Part model, mm, in its own coordinate system. Face numbers are marked on the shaded views. Round coordinates to 2 decimals unless told otherwise and drop trailing zeros. Write each loop counter-clockwise with the first axis right and the second up, starting at its lowest first coordinate (ties: lowest second). Pieces come first, ordered by that corner, then holes.
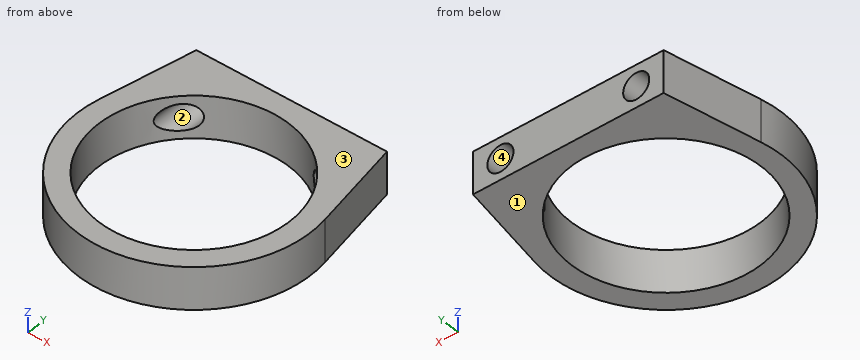
Autodesk Inventor part; units mm, degrees
ref_plane "YZ Plane" through (0, 0, 0) normal (1, 0, 0) x (0, 1, 0)
ref_plane "XZ Plane" through (0, 0, 0) normal (0, 1, 0) x (-1, 0, 0)
ref_plane "XY Plane" through (0, 0, 0) normal (0, 0, 1) x (1, 0, 0)
sketch "Sketch1" plane through (0, 0, 0) normal (0, 0, 1) x (1, 0, 0)
  circle A0 centre (0, 0) radius 9
  circle A1 centre (0, 0) radius 11
  line L0 (-9.125, 11) -> (9.125, 11)
  line L1 (0, 0) -> (0, 11) construction
  line L2 (-9.125, 11) -> (-10.8107, 2.0321)
  line L3 (9.125, 11) -> (10.8107, 2.0321)
  dimension "d0" = 18
  dimension "d1" = 22
  dimension "d2" = 18.25
extrude "Extrusion1" add sketch "Sketch1" along normal blind 4
sketch "Sketch2" plane through (-9.125, 11, 0) normal (0, 1, 0) x (1, 0, 0)
  line L0 (18.25, -4) -> (0, -4) construction
  line L1 (9.125, -4) -> (9.125, 0) construction
  line L2 (9.125, -2) -> (2.625, -2) construction
  line L3 (2.625, -2) -> (15.625, -2) construction
  circle A0 centre (2.625, -2) radius 1.25
  circle A1 centre (15.625, -2) radius 1.25
  dimension "d5" = 6.5
  dimension "d6" = 13
  dimension "d7" = 2.5
  dimension "d8" = 2.5
extrude "Extrusion2" cut sketch "Sketch2" against normal blind 11
thread "Thread1"
thread "Thread2"
equation "\"d6\" = 2 * d5"
properties part number "Tarot_12mm_Mount" material "Aluminum 6061"
Q1. Drop flat-ended pins along their axis: pin 1 (2 mm diameter, centred on x = -6.5, z = 2, fed in from -Y); pin 2 (12 mm diameter, centred on x = 5, y = -4, fed in from -Z). Give the stop position or say it passes through.
Values follow:
pin 1: stops at y = -9.53
pin 2: stops at z = 0
Q2. Cut at C-C on z = 1.6. Write the cut outline in (x, y) (3 decimals), plus the area to 3 significant figures.
Values follow:
outline: (-10.811, 2.032) arc R11 ccw (long way) to (10.811, 2.032) - (9.125, 11) - (7.684, 11) - (7.684, 4.685) arc R9 cw (long way) to (-7.684, 4.685) - (-7.684, 11) - (-9.125, 11) - close; (-5.316, 7.262) arc R9 cw to (5.316, 7.262) - (5.316, 11) - (-5.316, 11) - close
area: 136 mm2
Q3. Cut at A-A on y = 0. Write the cut outline in (x, z).
Values follow:
outline: (-11, 0) - (-9, 0) - (-9, 4) - (-11, 4) - close; (9, 0) - (11, 0) - (11, 4) - (9, 4) - close
Q4. Wall check: L1, parallel to Z at x = -6.5, y = 6.5; L2, parallel to Y at x = 0.5, z = 3.15; L3, parallel to X at y = -7, z = 1.95. Give the ranges that are in metal, low to high.
Values follow:
L1: z = 0 to 0.75, 3.25 to 4
L2: y = -10.99 to -8.99, 8.99 to 11
L3: x = -8.49 to -5.66, 5.66 to 8.49
Q5. Cut at D-D on x = -6.5. Write the cut outline in (y, z), plus the area to 3 significant figures.
Values follow:
outline: (-8.87, 0) - (-6.22, 0) - (-6.22, 4) - (-8.87, 4) - close; (6.22, 0) - (11, 0) - (11, 0.75) - (6.22, 0.75) - close; (6.22, 3.25) - (11, 3.25) - (11, 4) - (6.22, 4) - close
area: 17.8 mm2
Q6. Mould opens along Z. For the marked faces 1, 2, 3 and 4 say: +Z half, -Z half, draft (parallel to the pull), parting line (faces both ways), or undercut.
Values follow:
face 1: -Z half
face 2: undercut
face 3: +Z half
face 4: undercut
